from build123d import *

# Parameters (mm, degrees)
SKETCH_1_W          = 79
SKETCH_1_H          = 20
SKETCH_1_R          = 2.5
EXTRUDE_1_DEPTH     = 8
SKETCH_1_3_R        = 4.5
CUT_EXTRUDE_1_DEPTH = 5.2
SKETCH_1_4_R        = 4.5
CUT_EXTRUDE_2_DEPTH = 5.2


with BuildPart() as part:
    # 草图1 → 凸台-拉伸1 (new body)
    with BuildSketch(Plane.XY):
        with Locations((-19.987727126, 36.540514884)):
            Rectangle(SKETCH_1_W, SKETCH_1_H)
        with Locations((-40.737727126, 36.540514884)):
            Circle(SKETCH_1_R, mode=Mode.SUBTRACT)
        with Locations((-53.487727126, 36.540514884)):
            Circle(SKETCH_1_R, mode=Mode.SUBTRACT)
        with Locations((13.512272874, 36.540514884)):
            Circle(SKETCH_1_R, mode=Mode.SUBTRACT)
        with Locations((0.762272874, 36.540514884)):
            Circle(SKETCH_1_R, mode=Mode.SUBTRACT)
    extrude(amount=EXTRUDE_1_DEPTH)

    # 草图1<3> → 切除-拉伸1 (cut)
    with BuildSketch(Plane.XY):
        with Locations((0.762272874, 36.540514884)):
            Circle(SKETCH_1_3_R)
    extrude(amount=CUT_EXTRUDE_1_DEPTH, mode=Mode.SUBTRACT)

    # 草图1<4> → 切除-拉伸2 (cut)
    with BuildSketch(Plane.XY):
        with Locations((-40.737727126, 36.540514884)):
            Circle(SKETCH_1_4_R)
    extrude(amount=CUT_EXTRUDE_2_DEPTH, mode=Mode.SUBTRACT)


solid = part.part
Part model, mm, in its own coordinate system. A direction names the side the tool comes from. Coordinates: 2 decimals unless noted, no trailing zeros. Order: outer loops, then holes, each group sorted by start corner. A loop starts at its lowest first (then second) coordinate and runs counter-clockwise, first axis right, second up. Notation, with made-up numbers: M 0,-10 L 25,-10 A23 cw 25,6 Z; hole C 74,-18.5 d11. An arc over 180 degrees is marked long. Use a Markdown table: item, result.
(1) Probe L1, parallel to X at y = 36.75, z = 6; L2, parallel to Y at x = 4.5, z = 4.25; L3, parallel to X at y = 32.5, z = 0.5. List the from-to ranges inside material, lowest first.
A:
| item | result |
|---|---|
| L1 | x = -59.49 to -55.98, -51 to -43.23, -38.25 to -1.73, 3.25 to 11.02, 16 to 19.51 |
| L2 | y = 26.54 to 34.03, 39.05 to 46.54 |
| L3 | x = -59.49 to -42.72, -38.76 to -1.22, 2.74 to 19.51 |
(2) Cut at A-A on x = 2. Write the cut outline in (y, z).
A:
| item | result |
|---|---|
| outline | M 26.54,0 L 32.21,0 L 32.21,5.2 L 34.37,5.2 L 34.37,8 L 26.54,8 Z; M 38.71,5.2 L 40.87,5.2 L 40.87,0 L 46.54,0 L 46.54,8 L 38.71,8 Z |
(3) Pull direction Y, two halves, no side cores. Call faces 1 (the flat face through (-21, 37, 0)), 2 (the flat face through (-21, 46.541, 4)), 3 (the cylindrical face through (-38.66, 32.55, 2.56)): released by +Y, released by -Y, zero draft, split by the parting line, or undercut.
A:
| item | result |
|---|---|
| face 1 | zero draft |
| face 2 | released by +Y |
| face 3 | undercut |
(4) Cut at D-D on x = 14. Write the cut outline in (y, z), then the cut area to 3 significant figures.
A:
| item | result |
|---|---|
| outline | M 26.54,0 L 34.09,0 L 34.09,8 L 26.54,8 Z; M 38.99,0 L 46.54,0 L 46.54,8 L 38.99,8 Z |
| area | 121 mm^2 |
(5) Cut at B-B on z = 4. Write the cut outline in (x, y), then the cut area to 3 significant figures.
A:
| item | result |
|---|---|
| outline | M -59.49,26.54 L 19.51,26.54 L 19.51,46.54 L -59.49,46.54 Z; hole C -53.49,36.54 d5; hole C -40.74,36.54 d9; hole C 0.76,36.54 d9; hole C 13.51,36.54 d5 |
| area | 1,410 mm^2 |
(6) Flat gauge pins, fed straight in: pin 1 (6 mm diameter, centred on x = -40.74, y = 36.54, fed in from -Z); pin 2 (3 mm diameter, centred on x = 0.76, y = 36.54, fed in from +Z). Where does each tip first touch, or does it go through?
A:
| item | result |
|---|---|
| pin 1 | stops at z = 5.2 |
| pin 2 | passes through |
(7) Cut at C-C on x = -37.5. Write the cut outline in (y, z).
A:
| item | result |
|---|---|
| outline | M 26.54,0 L 33.42,0 L 33.42,5.2 L 39.67,5.2 L 39.67,0 L 46.54,0 L 46.54,8 L 26.54,8 Z |
(8) Tool access for faces 4 (the flat face through (3, 35, 5.2)), 5 (the flat face through (-59.488, 36, 4)): list every direction of +Z, -Z, +X, -X, +Y, -Y with a clear straight run to the whole face (end or side of a thin tool).
A:
| item | result |
|---|---|
| face 4 | -Z |
| face 5 | +Z, -Z, -X, +Y, -Y |
